Could you check a few things on this drawing? It's one solid part, dimensions in mm from its lowest x, y, z. A direction names the side the tool comes from. Round coordinates to 2 decimals unless told otherwise and drop trailing zeros. Order: outer loops, then holes, each group sorted by start corner. A loop starts at its lowest first (then second) coordinate and runs counter-clockwise, first axis right, second up. Notation, with made-up numbers: M 84,-26 L 127,-26 A16 cw 127,-22 Z; hole C -22.5,-18 d1. An arc over 180 degrees is marked long. Answer as CSV lines item,"result". Start each with the question number.
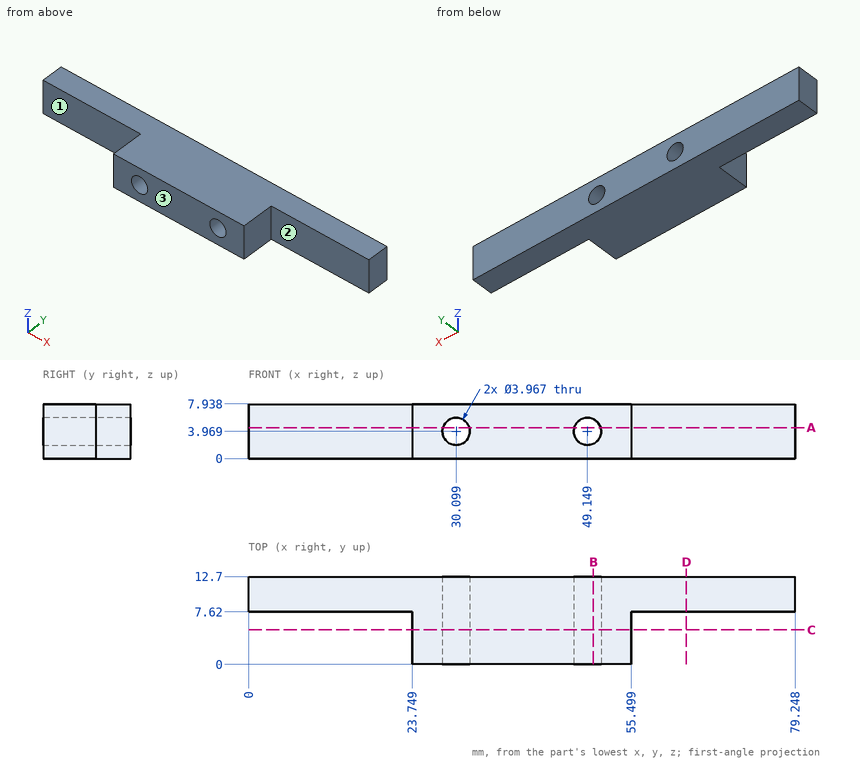
Item 1: If we section it at A-A on z = 4.5: Please give me the cut outline in (x, y).
Item 2: If we section it at D-D on x = 63.5: Please give me the cut outline in (y, z).
Item 3: Which directions (+Z, -Z, +X, -X, +Y, -Y) give clear straight access to the entire face, cutting with the end or side of a thin tool? Please do the marked faces 1, 2 and 3.
Item 4: For P1, Ø1, axis at y = 1.5, z = 4, coming from the +X side; P2, Ø3, axis at y = 5, z = 4, coming from the -X side; P3, Ø3, axis at x = 30.1, z = 3.97, coming from the +Y side; P4, Ø4, axis at x = 17.5, z = 2.5, coming from the -Y side, each with a flat end and sliding along its axis, tell me the tip position at first contact or that it passes through.
Item 5: If we section it at B-B on x = 50: Please give me the cut outline in (y, z).
Item 6: If we section it at C-C on y = 5: Count the separate pieces of the cut face and the enclosed holes in it, and give its area (3 significant figures).
Item 7: If I drill on line 1 along X through (y, z) = (9.5, 3.75); line 2 along X through (y, z) = (4.25, 3.75); line 3 along Y through (x, z) = (5.5, 5.25), over which ranges is the centre line in solid material (lowest first)?
Geometry says:
1,outline,"M 0,7.62 L 23.75,7.62 L 23.75,0 L 28.19,0 L 28.19,12.7 L 0,12.7 Z; M 32.01,0 L 47.24,0 L 47.24,12.7 L 32.01,12.7 Z; M 51.06,0 L 55.5,0 L 55.5,7.62 L 79.25,7.62 L 79.25,12.7 L 51.06,12.7 Z"
2,outline,"M 7.62,0 L 12.7,0 L 12.7,7.94 L 7.62,7.94 Z"
3,face 1,"+Z, -Z, -X, -Y"
3,face 2,"+Z, -Z, +X, -Y"
3,face 3,"+Z, -Z, +X, -X, -Y"
4,P1,"x = 55.5"
4,P2,"x = 23.75"
4,P3,"through"
4,P4,"y = 7.62"
5,outline,"M 0,0 L 12.7,0 L 12.7,2.18 L 0,2.18 Z; M 0,5.76 L 12.7,5.76 L 12.7,7.94 L 0,7.94 Z"
6,separate pieces,"1"
6,enclosed holes,"2"
6,area,"227 mm²"
7,line 1,"0 to 28.13, 32.07 to 47.18, 51.12 to 79.25"
7,line 2,"23.75 to 28.13, 32.07 to 47.18, 51.12 to 55.5"
7,line 3,"7.62 to 12.7"
